```python
from build123d import *

# Parameters (mm, degrees)
F0_W     = 70.196364
F0_H     = 41.332727
F1_DEPTH = 25.4
F2_R     = 11.06405
F3_DEPTH = 12.7
F5_DEPTH = 58.674


with BuildPart() as f1:
    # F0 (on Top) → F1 (new body)
    with BuildSketch(Plane.XY):
        with Locations((6.696364, -2.540001)):
            Rectangle(F0_W, F0_H)
    extrude(amount=F1_DEPTH)

    # F2 (on face) → F3 (join)
    with BuildSketch(Plane.XY.offset(25.4)):
        Circle(F2_R)
    extrude(amount=F3_DEPTH)

    # F4 (on face) → F5 (cut)
    with BuildSketch(Plane.XZ.offset(23.206364)):
        Polygon((11.06405, 38.1), (-11.06405, 38.1), (11.06405, 31.75), align=None)
    extrude(amount=-F5_DEPTH, mode=Mode.SUBTRACT)


solid = f1.part
```
The listing builds one solid part. Answer for the finished solid, in the listing's coordinates (mm). A direction names the side the tool comes from. Coordinates: 2 decimals unless noted, no trailing zeros. Write each loop counter-clockwise with the first axis right and the second up, starting at its lowest first coordinate (ties: lowest second). Pieces come first, ordered by that corner, then holes.
Q1. Section D-D, the plane x = -20 is taken. Write down the section's boundary in (y, z).
Returned:
outline: (-23.21, 0) - (18.13, 0) - (18.13, 25.4) - (-23.21, 25.4) - close
Q2. Section C-C, the plane z = 32.5 is taken. Write down the section's boundary in (x, y).
Returned:
outline: (8.45, -7.14) - (8.45, 7.14) arc R11.06 ccw (long way) to start
Q3. Section A-A, the plane y = 0 is taken. Write down the section's boundary in (x, z), then the cut area to 3 significant figures.
Returned:
outline: (-28.4, 0) - (41.79, 0) - (41.79, 25.4) - (11.06, 25.4) - (11.06, 31.75) - (-11.06, 38.1) - (-11.06, 25.4) - (-28.4, 25.4) - close
area: 1,990 mm2
Q4. Which of the six approach directions +Z, -Z, +X, -X, +Y, -Y give full straight-line access (tool end or side, diameter ignored) to faces 1 (the flat face through (6, -2, 0)), 2 (the cylindrical face through (-11.053, 0.486, 30.25))?
Returned:
face 1: -Z, +X, -X, +Y, -Y
face 2: +Z
Q5. Section B-B, the plane x = 0.5 is taken. Write down the section's boundary in (y, z), then the cut area to 3 significant figures.
Returned:
outline: (-23.21, 0) - (18.13, 0) - (18.13, 25.4) - (11.05, 25.4) - (11.05, 34.78) - (-11.05, 34.78) - (-11.05, 25.4) - (-23.21, 25.4) - close
area: 1,260 mm2
Q6. Find the intervals of material crossed by line 1 along Z through (x, y) = (22.5, 1); line 2 along X through (y, z) = (-0.5, 27.5); line 3 along Y through (x, z) = (-3, 27), in increasing order.
Returned:
line 1: z = 0 to 25.4
line 2: x = -11.05 to 11.05
line 3: y = -10.65 to 10.65
Q7. Given P1, Ø10, axis at x = 0.5, y = 7, coming from the +Z side; P2, Ø12, axis at x = -17.5, y = 13, coming from the +Z side; P3, Ø5, axis at y = 7.5, z = 32.5, coming from the -X side, each flat-ended and moving along its own axis, determine where each tip first touches the part or whether it passes through.
Returned:
P1: stops at z = 36.22
P2: stops at z = 25.4
P3: stops at x = -9.87
